from build123d import *

# Parameters (mm, degrees)
ESQUISSE1_W             = 15
ESQUISSE1_H             = 20
BOSS_EXTRU_1_DEPTH      = 1.5
ENL_V_MAT_EXTRU_1_REACH = 14.59
ESQUISSE2_R             = 1.5
ESQUISSE3_W             = 2
ESQUISSE3_H             = 20
BOSS_EXTRU_2_DEPTH      = 8
ESQUISSE4_W             = 4
ESQUISSE4_H             = 4
BOSS_EXTRU_3_DEPTH      = 1


with BuildPart() as part:
    # Esquisse1 → Boss.-Extru.1 (new body)
    with BuildSketch(Plane(origin=(0, 0, 0), x_dir=(1, 0, 0), z_dir=(0, 1, 0))):
        Rectangle(ESQUISSE1_W, ESQUISSE1_H)
    extrude(amount=BOSS_EXTRU_1_DEPTH)

    # Esquisse2 → Enlèv. mat.-Extru.1 (cut, up to next)
    with BuildSketch(Plane(origin=(0, 1.5, 0), x_dir=(1, 0, 0), z_dir=(0, 1, 0)), mode=Mode.PRIVATE) as enl_v_mat_extru_1_sk1:
        with Locations(Location((5.5, 7.5, 0), (0, 0, 270))):
            Circle(ESQUISSE2_R)
    enl_v_mat_extru_1_tool1 = extrude(enl_v_mat_extru_1_sk1.sketch, amount=-ENL_V_MAT_EXTRU_1_REACH, mode=Mode.PRIVATE) & part.part
    enl_v_mat_extru_1 = enl_v_mat_extru_1_tool1.solids().sort_by_distance((5.5, 1.5, -7.5))[0]
    add(enl_v_mat_extru_1, mode=Mode.SUBTRACT)

    # Symétrie1: Enlèv. mat.-Extru.1 across plane
    add(enl_v_mat_extru_1.mirror(Plane.XY), mode=Mode.SUBTRACT)

    # Esquisse3 → Boss.-Extru.2 (add)
    with BuildSketch(Plane(origin=(0, 1.5, 0), x_dir=(1, 0, 0), z_dir=(0, 1, 0))):
        with Locations((-6.5, 0)):
            Rectangle(ESQUISSE3_W, ESQUISSE3_H)
    extrude(amount=BOSS_EXTRU_2_DEPTH)

    # Esquisse4 → Boss.-Extru.3 (add)
    with BuildSketch(Plane(origin=(0, 1.5, 0), x_dir=(1, 0, 0), z_dir=(0, 1, 0))):
        with Locations((1, 0)):
            Rectangle(ESQUISSE4_W, ESQUISSE4_H)
    extrude(amount=BOSS_EXTRU_3_DEPTH)


solid = part.part
Can you work these out from the model? Positions are in its coordinate system, mm. A direction names the side the tool comes from. Coordinates: 2 decimals unless noted, no trailing zeros. Loops run counter-clockwise (first coordinate to the right, second up) from the corner with the lowest first, then second, coordinate; pieces in that order, holes last. Notation, with made-up numbers: (-39, 88.25) - (-25, 88.25) arc R14 cw to (-25, 95.25) - close; hole circle Ø3 at (-35, -35.5). An arc over 180 degrees is marked (long way). Answer as a JSON object with one key per item and string values. Group by question number.
Item 1: For pin 1 (0.8 mm diameter, centred on x = 0.5, y = 2, fed in from -Z); pin 2 (4 mm diameter, centred on y = 7, z = -2.5, fed in from +X); pin 3 (0.8 mm diameter, centred on y = 2, z = -0.5, fed in from +X); pin 4 (1.8 mm diameter, centred on x = 5.5, z = -7.5, fed in from -Y), each with a flat end and sliding along its axis, tell me the tip position at first contact or that it passes through.
Item 2: If we mould it in two halves opening along X, with no side actions, what happens to faces 4 (the face through (-7.5, 5, 0)), 5 (the face through (3, 2, 0)), 6 (the face through (-3, 1, 10)), 7 (the face through (5.57, 0.76, 9))? For each: released by +X, released by -X, zero draft, split by the parting line, or undercut.
Item 3: If we section it at D-D (x = -0.25): List the corners of the cut face in (y, z) for me, plus the area to 3 significant figures.
Item 4: On a 3-axis mill with a long thin cutter (end or side, diameter ignored), from which of +Z, -Z, +X, -X, +Y, -Y can I reach the whole of each face in a straight line? I mean faces 1 (the face through (-1, 2, 0)), 2 (the face through (1, 2.5, 0)), 3 (the face through (1, 2, -2)). Say none if no direction works.
Item 5: If we section it at B-B (z = -7.5): List the corners of the cut face in (x, y) for me, plus the area to 3 significant figures.
Item 6: If I drill on L1, parallel to X at y = 0.35, z = 7.5; L2, parallel to X at y = 7.25, z = -6.75; L3, parallel to Y at x = 6, z = 1.5, over which ranges is the centre line in solid material (lowest first)? Write a range as from..to.
Item 7: If we section it at A-A (x = 5.5): List the corners of the cut face in (y, z) for me, plus the area to 3 significant figures.
Item 8: If we section it at C-C (y = 2): List the corners of the cut face in (x, z) for me, plus the area to 3 significant figures.
Returned:
{
 "1": {"pin 1": "stops at z = -2", "pin 2": "stops at x = -5.5", "pin 3": "stops at x = 3", "pin 4": "passes through"},
 "2": {"face 4": "released by -X", "face 5": "released by +X", "face 6": "zero draft", "face 7": "undercut"},
 "3": {"outline": "(0, -10) - (1.5, -10) - (1.5, -2) - (2.5, -2) - (2.5, 2) - (1.5, 2) - (1.5, 10) - (0, 10) - close", "area": "34.0 mm²"},
 "4": {"face 1": "+Z, -Z, +Y", "face 2": "+Z, -Z, +X, +Y", "face 3": "-Z, +X, +Y"},
 "5": {"outline": "(-7.5, 0) - (4, 0) - (4, 1.5) - (-5.5, 1.5) - (-5.5, 9.5) - (-7.5, 9.5) - close; (7, 0) - (7.5, 0) - (7.5, 1.5) - (7, 1.5) - close", "area": "34.0 mm²"},
 "6": {"L1": "x = -7.5..4, 7..7.5", "L2": "x = -7.5..-5.5", "L3": "y = 0..1.5"},
 "7": {"outline": "(0, -10) - (1.5, -10) - (1.5, -9) - (0, -9) - close; (0, -6) - (1.5, -6) - (1.5, 6) - (0, 6) - close; (0, 9) - (1.5, 9) - (1.5, 10) - (0, 10) - close", "area": "21.0 mm²"},
 "8": {"outline": "(-7.5, -10) - (-5.5, -10) - (-5.5, 10) - (-7.5, 10) - close; (-1, -2) - (3, -2) - (3, 2) - (-1, 2) - close", "area": "56.0 mm²"}
}
